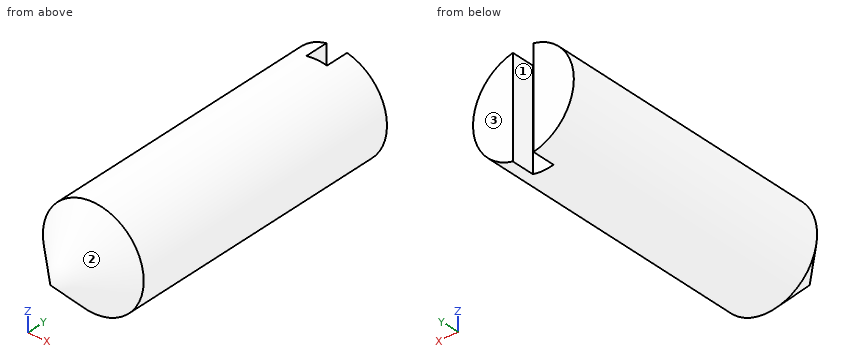
Autodesk Fusion 360 part; units mm, degrees
sketch "Sketch1" plane through (0, 0, 0) normal (0, 1, 0) x (1, 0, 0)
  circle A0 centre (0, 0) radius 3
  dimension "d1" = 6
extrude "Extrude1" add sketch "Sketch1" along normal blind 20
chamfer "Chamfer1" distance 3 angle 45 1 edges at (-2.797, 0, 1.0848)
ref_plane "WorkPlane1" through (0, 0, 3) normal (0, 0, 1) x (1, 0, 0)
sketch "Sketch2" plane through (0, 0, 3) normal (0, 0, 1) x (1, 0, 0)
  line L0 (3, 20) -> (-3, 20)
  line L1 (0, 20) -> (0, 18.6)
  line L2 (0, 18.6) -> (0.625, 18.6)
  line L3 (0.625, 18.6) -> (0.625, 20)
  line L4 (0.625, 20) -> (-0.605, 20)
  line L5 (-0.605, 20) -> (-0.605, 18.6)
  line L6 (-0.605, 18.6) -> (0.625, 18.6)
  dimension "d6" = 1.4
  dimension "d7" = 0.625
  dimension "d8" = 1.23
  dimension "d9" = 1.4
extrude "Extrude2" cut sketch "Sketch2" against normal blind 7
Check sheet for the modelled part. Datum: model origin and axes. Units: mm. Face numbers are marked on the shaded views. Round coordinates to 2 decimals unless told otherwise and drop trailing zeros. Write each loop counter-clockwise with the first axis right and the second up, starting at its lowest first coordinate (ties: lowest second). Pieces come first, ordered by that corner, then holes. Notation, with made-up numbers: M -25,-19 L 23,-19 A31 cw 23,13 Z; hole C 6,63.5 d10. An arc over 180 degrees is marked long. Write item = value, one per line. Start each with the question number.
1. Release check for a two-part mould opening along X. For the marked faces 1, 2 and 3 record: pulls with the +X half, pulls with the -X half, needs draft (parallel to the pull), parting line crosses it, or undercut.
2. Section check A-A, the plane y = 4.5. Record the cut outline in (x, z).
3. Scan lines: line 1 (X direction, y = 19, z = 0.8) (3 decimals); line 2 (Y direction, x = 0.7, z = -1.5); line 3 (Y direction, x = -0.65, z = -0.9). Record each from-to range of solid material in increasing order. Write a range as [from, to].
4. Gauge pin test, flat ends, axial feed: pin 1 (0.6 mm diameter, centred on x = -0.5, z = 1, fed in from +Y); pin 2 (1.5 mm diameter, centred on x = 1, y = 17.5, fed in from -Z); pin 3 (0.7 mm diameter, centred on y = 19.5, z = 0.5, fed in from -X). Record the tip position at first contact, or that the pin passes through.
Results found:
q1.face_1 = undercut
q1.face_2 = parting line crosses it
q1.face_3 = needs draft
q2.outline = C 0,0 d6
q3.line_1 = [-2.891, -0.605], [0.625, 2.891]
q3.line_2 = [1.66, 20]
q3.line_3 = [1.11, 20]
q4.pin_1 = 20
q4.pin_2 = -2.99
q4.pin_3 = -3
